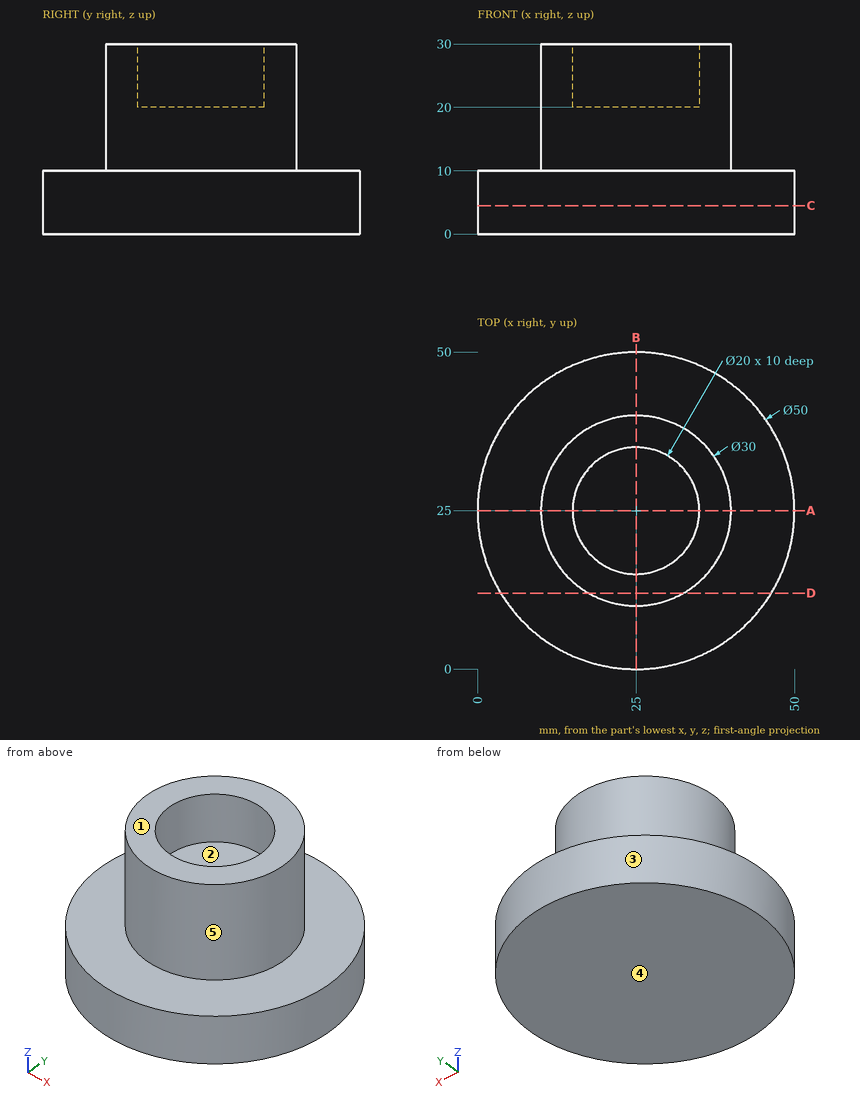
Drawing for the job (mm, zero at the part's lowest x, y, z). A direction names the side the tool comes from. Coordinates: 2 decimals unless noted, no trailing zeros. Write each loop counter-clockwise with the first axis right and the second up, starting at its lowest first coordinate (ties: lowest second). Pieces come first, ordered by that corner, then holes. Notation, with made-up numbers: (51, 18) - (66, 18) arc R21 cw to (66, 43) - close; hole circle Ø2 at (1.5, 76). An arc over 180 degrees is marked (long way). Write each question's results on one line, items separated by ' | '. Start each with the question number.
1) Probe line 1 along Y through (x, z) = (25, 27.75); line 2 along X through (y, z) = (27, 25.75); line 3 along Z through (x, y) = (25, 29). List the from-to ranges inside material, lowest first. Write a range as from..to.
2) Flat gauge pins, fed straight in: P1, Ø25, axis at x = 31.5, y = 27, coming from the +Z side; P2, Ø8, axis at x = 10, y = 43.5, coming from the +Z side; P3, Ø4, axis at y = 37.5, z = 22, coming from the +X side; P4, Ø8, axis at y = 30.5, z = 3.5, coming from the -X side. Where does each tip first touch, or does it go through?
3) Cut at D-D (y = 12). Write the cut outline in (x, z), then the cut area to 3 significant figures.
4) Cut at C-C (z = 4.5). Write the cut outline in (x, y), then the cut area to 3 significant figures.
5) Cut at A-A (y = 25). Write the cut outline in (x, z), then the cut area to 3 significant figures.
6) Mould opens along X. For the marked faces 1, 2 and 3 say: pulls with the +X half, pulls with the -X half, needs draft (parallel to the pull), parting line crosses it, or undercut.
7) 3-axis set-ups, long thin cutter, end or side, ignore diameter. For the marked faces 4 and 5: which of +Z, -Z, +X, -X, +Y, -Y reach the whole face in a straight line?
Returned:
1) line 1: 10..15, 35..40 | line 2: 10.13..15.2, 34.8..39.87 | line 3: 0..20
2) P1: z = 30 | P2: z = 10 | P3: x = 35.71 | P4: x = 0.05
3) outline: (3.65, 0) - (46.35, 0) - (46.35, 10) - (32.48, 10) - (32.48, 30) - (17.52, 30) - (17.52, 10) - (3.65, 10) - close | area: 726 mm^2
4) outline: circle Ø50 at (25, 25) | area: 1,960 mm^2
5) outline: (0, 0) - (50, 0) - (50, 10) - (40, 10) - (40, 30) - (35, 30) - (35, 20) - (15, 20) - (15, 30) - (10, 30) - (10, 10) - (0, 10) - close | area: 900 mm^2
6) face 1: needs draft | face 2: undercut | face 3: parting line crosses it
7) face 4: -Z, +X, -X, +Y, -Y | face 5: +Z
